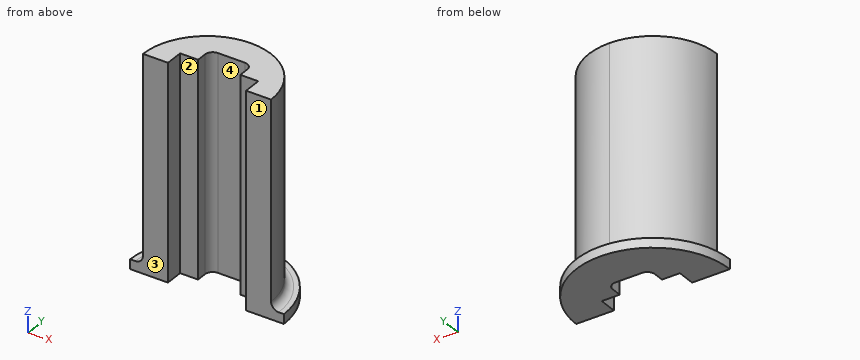
from build123d import *

# Parameters (mm, degrees)
F1_DEPTH = 41.75
F2_START = -38
F2_DEPTH = 3.75
F3_R     = 3


with BuildPart() as f1:
    # F0 (on Top) → F1 (new body, symmetric)
    with BuildSketch(Plane.XY):
        with BuildLine():
            Line((-25, -7), (-15.25, -7))
            Line((-15.25, -7), (-15.25, 0))
            Line((-15.25, 0), (-8.25, 0))
            Line((-8.25, 0), (-8.25, 7))
            Line((-8.25, 7), (0, 7))
            Line((0, 7), (0, 18))
            ThreePointArc((0, 18), (-17.6776695297, 10.6776695297), (-25, -7))
        make_face()
    extrude(amount=F1_DEPTH, both=True)

    # F0 (on Top) → F2 (join)
    with BuildSketch(Plane.XY.offset(F2_START)):
        with BuildLine():
            Line((-30, -7), (-25, -7))
            ThreePointArc((-25, -7), (-17.6776695297, 10.6776695297), (0, 18))
            Line((0, 18), (0, 23))
            ThreePointArc((0, 23), (-21.2132034356, 14.2132034356), (-30, -7))
        make_face()
    extrude(amount=-F2_DEPTH)

    # F3
    f3_edges = [f1.edges().sort_by_distance(p)[0] for p in [
        (-8.25, 7, 0),
        (-17.67767, 10.67767, -38),
    ]]
    fillet(f3_edges, radius=F3_R)

    # F4: F1 across plane


with BuildPart() as f1_1:
    add(f1.part)
    add(f1.part.mirror(Plane.YZ))


solid = f1_1.part
CAD build for the part. Positions are in the model's coordinates, mm. Face numbers are marked on the shaded views. A direction names the side the tool comes from. Give positions to 0.01 mm unless a question says otherwise; leave off trailing zeros. Write each loop counter-clockwise with the first axis right and the second up, starting at its lowest first coordinate (ties: lowest second). Pieces come first, ordered by that corner, then holes. Notation, with made-up numbers: M 82.25,-16.75 L 137.25,-16.75 A12 cw 137.25,-4.75 Z; hole C 44.25,-31 d10. An arc over 180 degrees is marked long. Put each result on its own line as item: value. Start each with the question number.
(1) Mould opens along X. For the marked faces 3 and 4 say: +X half, -X half, draft (parallel to the pull), parting line (faces both ways), or undercut.
(2) Band-saw the part on A-A, the plane z = 17. Write the cut outline in (x, y).
(3) Which spindle directions (+Z, -Z, +X, -X, +Y, -Y) get a long thin tool onto all of the face, cutting with end or side? Do the marked faces 1 and 2. Say none if no direction does.
(4) Flat gauge pins, fed straight in: pin 1 Ø2 at (y, z) = (10.5, 29.5) entering from -X; pin 2 Ø7.5 at (y, z) = (-3, 11) entering from -X; pin 3 Ø2 at (y, z) = (-2.5, 14) entering from +X. Where does each tip first touch, or does it go through?
(5) Probe L1, parallel to X at y = 5.5, z = -12; L2, parallel to Z at x = 12, y = 18; L3, parallel to X at y = 3, z = 19. List the from-to ranges inside material, lowest first.
Response values:
1. face 3: draft
1. face 4: undercut
2. outline: M -25,-7 L -15.25,-7 L -15.25,0 L -8.25,0 L -8.25,4 A3 cw -5.25,7 L 5.25,7 A3 cw 8.25,4 L 8.25,0 L 15.25,0 L 15.25,-7 L 25,-7 A25 ccw Z
3. face 1: +Z, -Z, +X, -X, -Y
3. face 2: +Z, -Z, -Y
4. pin 1: stops at x = -18.78
4. pin 2: stops at x = -25
4. pin 3: stops at x = 24.75
5. L1: x = -21.65 to -7.85, 7.85 to 21.65
5. L2: z = -41.75 to -37.99
5. L3: x = -22.91 to -8.25, 8.25 to 22.91
